Build history of the part. All positions in model axes, mm. Round coordinates to 2 decimals unless told otherwise and drop trailing zeros. Write each loop counter-clockwise with the first axis right and the second up, starting at its lowest first coordinate (ties: lowest second). Pieces come first, ordered by that corner, then holes.
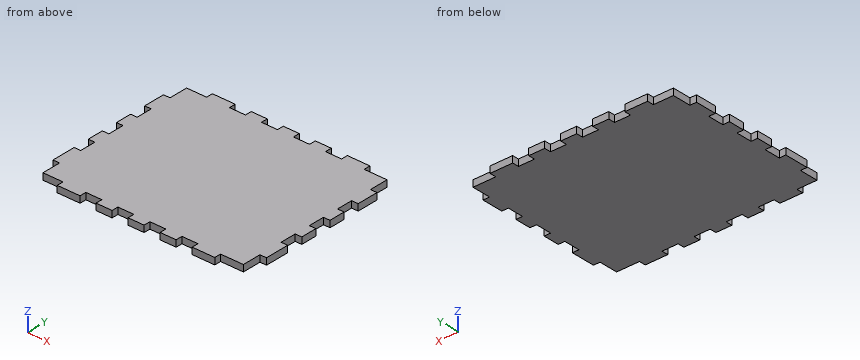
from build123d import *

# Parameters (mm, degrees)
F0_W     = 169.333316
F0_H     = 139.7
F1_DEPTH = 5.207
F2_W     = 5.207
F2_H     = 12.7
F2_W_2   = 12.7
F2_H_2   = 5.207
F3_DEPTH = 5.208


with BuildPart() as f1:
    # F0 (on Top) → F1 (new body)
    with BuildSketch(Plane.XY):
        Rectangle(F0_W, F0_H)
    extrude(amount=F1_DEPTH)

    # F2 (on face) → F3 (cut, through all)
    with BuildSketch(Plane.XY.offset(5.207)):
        Polygon((-79.459658, 49.73955), (-79.459658, 64.643), (-63.584658, 64.643), (-63.584658, 69.85), (-84.666658, 69.85), (-84.666658, 49.73955), align=None)
        with Locations((-82.063158, 26.456386)):
            Rectangle(F2_W, F2_H)
        with Locations((-82.063158, 1.056386)):
            Rectangle(F2_W, F2_H)
        with Locations((-82.063158, -24.343614)):
            Rectangle(F2_W, F2_H)
        Polygon((-79.459658, -49.743614), (-84.666658, -49.743614), (-84.666658, -69.85), (-63.584658, -69.85), (-63.584658, -64.643), (-79.459658, -64.643), align=None)
        with Locations((-39.13505, -67.2465)):
            Rectangle(F2_W_2, F2_H_2)
        with Locations((-13.73505, -67.2465)):
            Rectangle(F2_W_2, F2_H_2)
        with Locations((11.66495, -67.2465)):
            Rectangle(F2_W_2, F2_H_2)
        with Locations((37.06495, -67.2465)):
            Rectangle(F2_W_2, F2_H_2)
        Polygon((61.36005, -64.643), (61.36005, -69.85), (84.666658, -69.85), (84.666658, -49.743783), (79.459658, -49.743783), (79.459658, -64.643), align=None)
        with Locations((82.063158, -24.343783)):
            Rectangle(F2_W, F2_H)
        with Locations((82.063158, 1.056217)):
            Rectangle(F2_W, F2_H)
        Polygon((84.666658, 69.85), (61.36005, 69.85), (61.36005, 64.643), (79.459658, 64.643), (79.459658, 49.73955), (84.666658, 49.73955), align=None)
        with Locations((37.06495, 67.2465)):
            Rectangle(F2_W_2, F2_H_2)
        with Locations((11.66495, 67.2465)):
            Rectangle(F2_W_2, F2_H_2)
        with Locations((82.063158, 26.456217)):
            Rectangle(F2_W, F2_H)
        with Locations((-13.73505, 67.2465)):
            Rectangle(F2_W_2, F2_H_2)
        with Locations((-39.13505, 67.2465)):
            Rectangle(F2_W_2, F2_H_2)
    extrude(amount=-F3_DEPTH, mode=Mode.SUBTRACT)


solid = f1.part
1) Slice it at A-A (y = 22). Write the cut outline in (x, z), plus the area to 3 significant figures.
Results:
outline: (-79.46, 0) - (79.46, 0) - (79.46, 5.21) - (-79.46, 5.21) - close
area: 827 mm2
2) Wall check: L1, parallel to X at y = 5, z = 2.5; L2, parallel to Y at x = 62.5, z = 0.5. Give the ranges that are in metal, low to high.
Results:
L1: x = -79.46 to 79.46
L2: y = -64.64 to 64.64
3) Pin check, flat tips, straight feed: pin 1 Ø2.5 at (y, z) = (68.5, 1.5) entering from +X; pin 2 Ø2.5 at (x, z) = (14, 3.5) entering from -Y. Stop position of each tip, or through.
Results:
pin 1: stops at x = 61.36
pin 2: stops at y = -64.64
4) Slice it at B-B (x = -72). Write the cut outline in (y, z).
Results:
outline: (-64.64, 0) - (64.64, 0) - (64.64, 5.21) - (-64.64, 5.21) - close
